Here's how the part is built. I have some questions about the finished solid (model axes, mm). A direction names the side the tool comes from. Give positions to 0.01 mm unless a question says otherwise; leave off trailing zeros. Write each loop counter-clockwise with the first axis right and the second up, starting at its lowest first coordinate (ties: lowest second). Pieces come first, ordered by that corner, then holes. Notation, with made-up numbers: (25, -7.5) -> (56, -7.5) arc R12 cw to (56, 11.5) -> close; hole circle Ø8 at (-30, -40). An arc over 180 degrees is marked (long way). Use one line per item in the form item = value.
```python
from build123d import *

# Parameters (mm, degrees)
BOSS_EXTRUDE1_DEPTH = 40
CHAMFER1_SIZE       = 20
CHAMFER2_SIZE       = 30
SKETCH2_R           = 3.25
CUT_EXTRUDE1_DEPTH  = 32
CUT_EXTRUDE5_START  = 5
SKETCH2_3_R         = 3.25
CUT_EXTRUDE5_DEPTH  = 32
SKETCH5_R           = 1.65
CUT_EXTRUDE2_DEPTH  = 109.988531507
SKETCH6_R           = 3
CUT_EXTRUDE3_DEPTH  = 76.5
SKETCH7_R           = 1.5
CUT_EXTRUDE4_DEPTH  = 10
SKETCH8_R           = 1.5
CUT_EXTRUDE6_DEPTH  = 76.478231012
CUT_EXTRUDE7_DEPTH  = 93.643917135
SKETCH10_R          = 1.5
CUT_EXTRUDE8_DEPTH  = 5


with BuildPart() as part:
    # Sketch1 → Boss-Extrude1 (new body)
    with BuildSketch(Plane.XY):
        Polygon((10, 57.5), (15, 57.5), (15, 30.75), (93.5, 30.75), (93.5, 0), (78.5, 0), (78.5, 23.75), (10, 23.75), align=None)
    boss_extrude1 = extrude(amount=-BOSS_EXTRUDE1_DEPTH)

    # Mirror1: Boss-Extrude1 across plane
    add(boss_extrude1.mirror(Plane(origin=(78.5, 0, -40), x_dir=(0, 0, 1), z_dir=(0, -1, 0))))

    # Chamfer1
    chamfer1_edges = [part.edges().sort_by_distance(p)[0] for p in [
        (78.5, 23.75, -20),
        (78.5, -23.75, -20),
    ]]
    chamfer(chamfer1_edges, length=CHAMFER1_SIZE)

    # Chamfer2
    # the kernel refuses this chamfer: 30 mm, written as the material it adds along each edge
    with BuildSketch(Plane(origin=(15, 30.75, 0), x_dir=(0.9996219169112968, -0.02749587661058632, 0), z_dir=(0, 0, -1))) as chamfer2_piece_1_section:
        Polygon((CHAMFER2_SIZE * 0.999621916911, -CHAMFER2_SIZE * 0.0274958766106), (-CHAMFER2_SIZE * 0.0274958766106, -CHAMFER2_SIZE * 0.999621916911), (0, 0), align=None)
    chamfer2_piece_1 = extrude(amount=40, mode=Mode.PRIVATE)
    chamfer2_piece_1 = split(chamfer2_piece_1, bisect_by=Plane(origin=(25.097042378, 57.5, -20), z_dir=(0, -1, 0)), keep=Keep.TOP, mode=Mode.PRIVATE)
    add(chamfer2_piece_1)
    with BuildSketch(Plane(origin=(15, -30.75, 0), x_dir=(-0.02749587661058655, -0.9996219169112968, 0), z_dir=(0, 0, -1))) as chamfer2_piece_2_section:
        Polygon((CHAMFER2_SIZE * 0.999621916911, -CHAMFER2_SIZE * 0.0274958766106), (-CHAMFER2_SIZE * 0.0274958766106, -CHAMFER2_SIZE * 0.999621916911), (0, 0), align=None)
    chamfer2_piece_2 = extrude(amount=40, mode=Mode.PRIVATE)
    chamfer2_piece_2 = split(chamfer2_piece_2, bisect_by=Plane(origin=(25.097042378, -57.5, -20), z_dir=(0, 1, 0)), keep=Keep.TOP, mode=Mode.PRIVATE)
    add(chamfer2_piece_2)

    # Sketch2 → Cut-Extrude1 (cut)
    with BuildSketch(Plane(origin=(51.601375419, 0, -14.7964563), x_dir=(0, -1, 0), z_dir=(0.9612616959383188, 0, -0.27563735581699983))):
        with Locations(Location((0, -10.918329477, 0), (0, 0, 270))):
            Circle(SKETCH2_R)
    extrude(amount=CUT_EXTRUDE1_DEPTH, mode=Mode.SUBTRACT)

    # Sketch2<3> → Cut-Extrude5 (cut)
    with BuildSketch(Plane(origin=(51.601375419, 0, -14.7964563), x_dir=(0, -1, 0), z_dir=(0.9612616959383188, 0, -0.27563735581699983)).offset(CUT_EXTRUDE5_START)):
        with Locations(Location((0, 6.865011898, 0), (0, 0, 270))):
            Circle(SKETCH2_3_R)
    extrude(amount=CUT_EXTRUDE5_DEPTH, mode=Mode.SUBTRACT)

    # Sketch5 → Cut-Extrude2 (cut, through all)
    with BuildSketch(Plane(origin=(93.5, 0, 0), x_dir=(0, 0, -1), z_dir=(1, 0, 0))):
        with Locations((31, -47.5)):
            Circle(SKETCH5_R)
        with Locations((9, -47.5)):
            Circle(SKETCH5_R)
        with Locations((9, 47.5)):
            Circle(SKETCH5_R)
        with Locations((31, 47.5)):
            Circle(SKETCH5_R)
    extrude(amount=-CUT_EXTRUDE2_DEPTH, mode=Mode.SUBTRACT)

    # Sketch6 → Cut-Extrude3 (cut)
    with BuildSketch(Plane(origin=(93.5, 0, 0), x_dir=(0, 0, -1), z_dir=(1, 0, 0))):
        with Locations(Location((31, -47.5, 0), (0, 0, 90))):
            Circle(SKETCH6_R)
        with Locations(Location((9, -47.5, 0), (0, 0, 90))):
            Circle(SKETCH6_R)
        with Locations(Location((31, 47.5, 0), (0, 0, 270))):
            Circle(SKETCH6_R)
        with Locations(Location((9, 47.5, 0), (0, 0, 270))):
            Circle(SKETCH6_R)
    extrude(amount=-CUT_EXTRUDE3_DEPTH, mode=Mode.SUBTRACT)

    # Sketch7 → Cut-Extrude4 (cut)
    with BuildSketch(Plane(origin=(93.5, 0, 0), x_dir=(0, 0, -1), z_dir=(1, 0, 0))):
        with Locations((20, -19.166666667)):
            Circle(SKETCH7_R)
        with Locations((20, 19.166666667)):
            Circle(SKETCH7_R)
    extrude(amount=-CUT_EXTRUDE4_DEPTH, mode=Mode.SUBTRACT)

    # Sketch8 → Cut-Extrude6 (cut, through all)
    with BuildSketch(Plane(origin=(51.601375419, 0, -14.7964563), x_dir=(0, -1, 0), z_dir=(0.9612616959383188, 0, -0.27563735581699983))):
        with Locations(Location((0, -10.918329477, 0), (0, 0, 270))):
            Circle(SKETCH8_R)
        with Locations(Location((0, 6.865011898, 0), (0, 0, 270))):
            Circle(SKETCH8_R)
    extrude(amount=CUT_EXTRUDE6_DEPTH, mode=Mode.SUBTRACT)

    # Sketch9 → Cut-Extrude7 (cut, through all)
    with BuildSketch(Plane(origin=(77.713455589, 0, -13.702978984), x_dir=(-0.17364817766693075, 0, -0.9848077530122081), z_dir=(0.9848077530122081, 0, -0.17364817766693075))):
        with BuildLine():
            Line((4.81351977, -13.75), (14.81351977, -13.75))
            Line((14.81351977, -13.75), (30.80281724, -13.75))
            Line((30.80281724, -13.75), (30.80281724, 13.75))
            Line((30.80281724, 13.75), (6.250897221, 13.75))
            Line((6.250897221, 13.75), (4.81351977, 13.75))
            ThreePointArc((4.81351977, 13.75), (-8.93648023, 0), (4.81351977, -13.75))
        make_face()
    extrude(amount=-CUT_EXTRUDE7_DEPTH, mode=Mode.SUBTRACT)

    # Sketch10 → Cut-Extrude8 (cut)
    with BuildSketch(Plane(origin=(0, 30.75, 0), x_dir=(1, 0, 0), z_dir=(0, 1, 0))):
        with Locations(Location((80.822063113, 29.543969578, 0), (0, 0, 270))):
            Circle(SKETCH10_R)
        with Locations(Location((57.677936887, 10.456030422, 0), (0, 0, 270))):
            Circle(SKETCH10_R)
    extrude(amount=-CUT_EXTRUDE8_DEPTH, mode=Mode.SUBTRACT)


solid = part.part
```
Q1. I want a section at C-C, the plane z = -2. Write out the boundary of the cut face in (x, y).
Result set:
outline = (10, -57.5) -> (18.25, -57.5) -> (45, -30.75) -> (93.5, -30.75) -> (93.5, 30.75) -> (45, 30.75) -> (18.25, 57.5) -> (10, 57.5) -> (10, 23.75) -> (58.5, 23.75) -> (78.5, 3.75) -> (78.5, -3.75) -> (58.5, -23.75) -> (10, -23.75) -> close
Q2. If we mould it in two halves opening along X, with no side actions, what happens to faces 1 (the face through (17, 46, -8)), 2 (the face through (22.64, -44.73, -32.15)), 3 (the face through (58, 25.75, -10)), 4 (the face through (78.5, 0, -3))? For each: +X half, -X half, draft (parallel to the pull), parting line (faces both ways), or undercut.
Result set:
face_1 = +X half
face_2 = draft
face_3 = undercut
face_4 = -X half
Q3. Will these pins go through, and if not, where does the flat tip stop? pin 1 Ø5 at (y, z) = (47.5, -31) entering from +X; pin 2 Ø12 at (y, z) = (13, -26.5) entering from -X; pin 3 Ø1.8 at (x, z) = (57.68, -10.46) entering from -Y.
Result set:
pin_1 = 17
pin_2 = 63.25
pin_3 = -30.75
Q4. Which directions (+Z, -Z, +X, -X, +Y, -Y) give clear straight access to the entire face, cutting with the end or side of a thin tool? Please do faces 5 (the face through (79.909, 28.285, -30.734)), 6 (the face through (72, 13.75, -29)), 7 (the face through (35, 23.75, -20)), 8 (the face through (22.64, -44.64, -8.1)).
Result set:
face_5 = +Y
face_6 = -X
face_7 = +Z, -Z, -X
face_8 = +X
Q5. I want a section at D-D, the plane y = 12.5. Write out the boundary of the cut face in (x, z), and give its area (3 significant figures).
Result set:
outline = (69.75, -11.37) -> (77.87, -12.8) -> (73.08, -40) -> (93.5, -40) -> (93.5, 0) -> (69.75, 0) -> close
area = 788 mm2
Q6. If I drill on line 1 along Y through (x, z) = (12, -31); line 2 along Y through (x, z) = (25, -9); line 3 along Y through (x, z) = (13.5, -24), over which ranges is the centre line in solid material (lowest first)? Write a range as from..to.
Result set:
line_1 = -57.5..-49.15, -45.85..-23.75, 23.75..45.85, 49.15..57.5
line_2 = -50.75..-50.5, -44.5..-23.75, 23.75..44.5, 50.5..50.75
line_3 = -57.5..-23.75, 23.75..57.5
Q7. I want a section at B-B, the plane x = 63. Write out the boundary of the cut face in (y, z).
Result set:
outline = (-30.75, -40) -> (-19.25, -40) -> (-19.25, 0) -> (-30.75, 0) -> close; (19.25, -40) -> (30.75, -40) -> (30.75, 0) -> (19.25, 0) -> close
Q8. I want a section at A-A, the plane y = 47.5. Write out the boundary of the cut face in (x, z).
Result set:
outline = (10, -40) -> (28.25, -40) -> (28.25, -34) -> (17, -34) -> (17, -32.65) -> (10, -32.65) -> close; (10, -29.35) -> (17, -29.35) -> (17, -28) -> (28.25, -28) -> (28.25, -12) -> (17, -12) -> (17, -10.65) -> (10, -10.65) -> close; (10, -7.35) -> (17, -7.35) -> (17, -6) -> (28.25, -6) -> (28.25, 0) -> (10, 0) -> close
